Verification items for this drawing (mm, ordinates from the low corner). A direction names the side the tool comes from. Coordinates: 2 decimals unless noted, no trailing zeros. Write each loop counter-clockwise with the first axis right and the second up, starting at its lowest first coordinate (ties: lowest second). Pieces come first, ordered by that corner, then holes. Notation, with made-up numbers: M -1,23.5 L 38,23.5 A17 ccw 38,30.5 Z; hole C 88.5,80.25 d3. An arc over 180 degrees is marked long. Put each result on its own line as item: value. Start each with the question number.
1) Set-up check for the marked faces 5, 6, 7, 8 and 9: record each of +Z, -Z, +X, -X, +Y, -Y from which the full face is reachable in a straight line by a thin tool's end or side.
2) Gauge pin test, flat ends, axial feed: pin 1 (4 mm diameter, centred on x = 17.5, z = 11, fed in from -Y) (3 decimals); pin 2 (4 mm diameter, centred on x = 14.5, z = 14.5, fed in from -Y); pin 3 (1 mm diameter, centred on x = 26, y = 21.5, fed in from +Z). Record the tip position at first contact, or that the pin passes through.
3) Scan lines: line 1 along X through (y, z) = (17, 14.5); line 2 along Z through (x, y) = (11, 28); line 3 along Y through (x, z) = (24.5, 13). Record each from-to range of solid material in increasing order.
4) Mould release check, pull along Y, two halves, no side actions. Record for the marked faces 1, 2, 3 and 4: released by +Y, released by -Y, zero draft, split by the parting line, or undercut.
5) Cross-section at B-B on z = 15.24. Count the separate pieces of the cut face and the enclosed holes in it, plus the area to 3 significant figures.
6) Cross-section at A-A on z = 4.5. Record the cut outline in (x, y), plus the area to 3 significant figures.
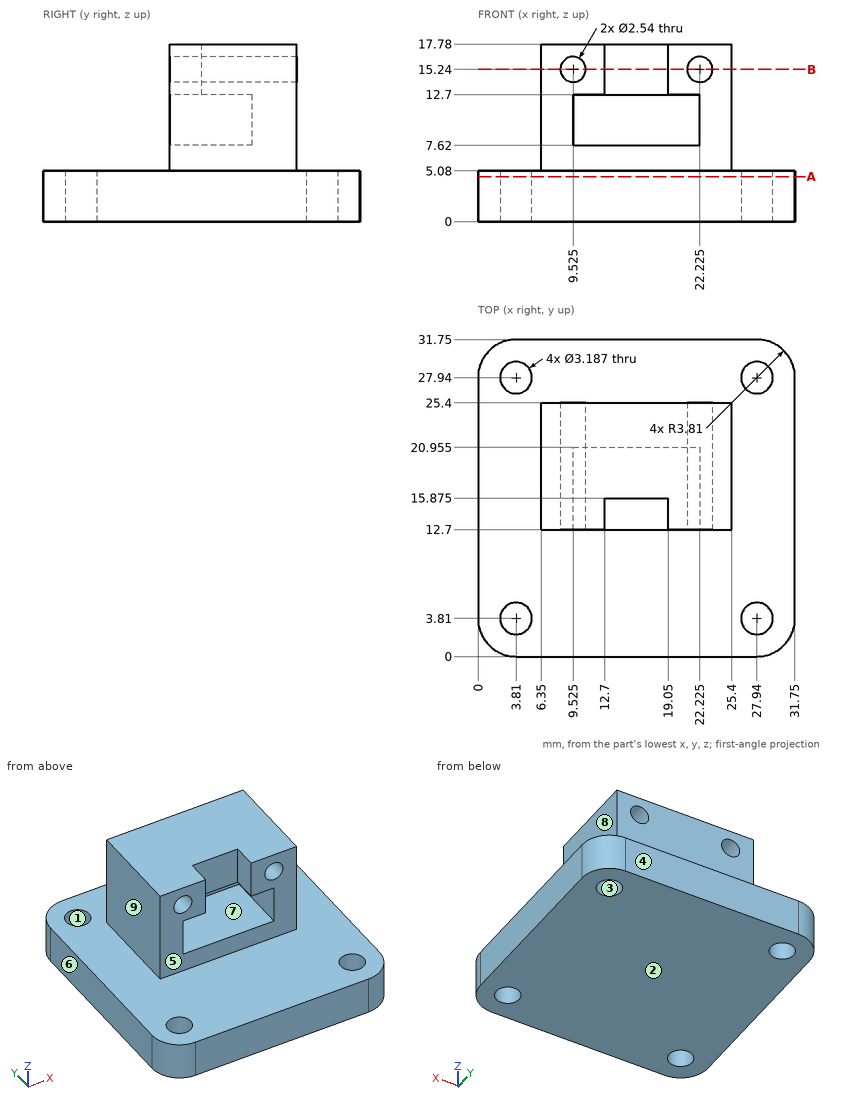
Answer key:
1. face 5: +Z, +X, -X, -Y
1. face 6: +Z, -Z, -X, +Y, -Y
1. face 7: -Y
1. face 8: +Z, +X, +Y, -Y
1. face 9: +Z, -X, +Y, -Y
2. pin 1: stops at y = 15.875
2. pin 2: stops at y = 12.7
2. pin 3: stops at z = 5.08
3. line 1: x = 6.35 to 8.49, 10.56 to 21.19, 23.26 to 25.4
3. line 2: z = 0 to 5.08
3. line 3: y = 12.7 to 25.4
4. face 1: undercut
4. face 2: zero draft
4. face 3: undercut
4. face 4: released by +Y
5. separate pieces: 3
5. enclosed holes: 0
5. area: 157 mm²
6. outline: M 0,3.81 A3.81 ccw 3.81,0 L 27.94,0 A3.81 ccw 31.75,3.81 L 31.75,27.94 A3.81 ccw 27.94,31.75 L 3.81,31.75 A3.81 ccw 0,27.94 Z; hole C 3.81,3.81 d3.19; hole C 3.81,27.94 d3.19; hole C 27.94,3.81 d3.19; hole C 27.94,27.94 d3.19
6. area: 964 mm²
